from build123d import *

# Parameters (mm, degrees)
F0_R     = 2
F1_DEPTH = 0.5


with BuildPart() as f1:
    # F0 (on Front) → F1 (new body, symmetric)
    with BuildSketch(Plane.XZ):
        with BuildLine():
            Line((-25.05, -3.9878), (0, -3.9878))
            ThreePointArc((0, -3.9878), (3.9878, 0), (0, 3.9878))
            Line((0, 3.9878), (-25.05, 3.9878))
            Line((-25.05, 3.9878), (-25.05, -3.9878))
        make_face()
        with Locations((-19.0556, 0)):
            Circle(F0_R, mode=Mode.SUBTRACT)
        with Locations((-11.9944, 0)):
            Circle(F0_R, mode=Mode.SUBTRACT)
        Circle(F0_R, mode=Mode.SUBTRACT)
    extrude(amount=F1_DEPTH, both=True)


solid = f1.part
Geometry: final body of the model. Coordinates: model frame, mm. Round coordinates to 2 decimals unless told otherwise and drop trailing zeros. Loops run counter-clockwise (first coordinate to the right, second up) from the corner with the lowest first, then second, coordinate; pieces in that order, holes last. Notation, with made-up numbers: M 5.5,-2 L 64.5,-2 A21 ccw 64.5,31 Z; hole C -37,81 d10. An arc over 180 degrees is marked long. One line per question, with ' | ' between items.
(1) Cut plane C-C on z = -1.25. Return the cut outline in (x, y).
Check result:
outline: M -25.05,-0.5 L -20.62,-0.5 L -20.62,0.5 L -25.05,0.5 Z; M -17.49,-0.5 L -13.56,-0.5 L -13.56,0.5 L -17.49,0.5 Z; M -10.43,-0.5 L -1.56,-0.5 L -1.56,0.5 L -10.43,0.5 Z; M 1.56,-0.5 L 3.79,-0.5 L 3.79,0.5 L 1.56,0.5 Z
(2) Pull-direction query (X, two-part tool) for faces 1 (the cylindrical face through (0, 0, -2)), 2 (the flat face through (-13, 0, -3.988)), 3 (the cylindrical face through (3.987, -0.007, -0.088)); classes: +X half, -X half, draft (parallel to the pull), parting line (faces both ways), or undercut.
Check result:
face 1: undercut | face 2: draft | face 3: +X half
(3) Material intervals for line 1 along X through (y, z) = (-0.15, -0.5); line 2 along Z through (x, y) = (-19, -0.2); line 3 along Z through (x, y) = (-1, -0.1), sorted ascending. Write a range as from..to.
Check result:
line 1: x = -25.05..-20.99, -17.12..-13.93, -10.06..-1.94, 1.94..3.96 | line 2: z = -3.99..-2, 2..3.99 | line 3: z = -3.99..-1.73, 1.73..3.99
(4) Cut plane A-A on y = 0.2. Return the cut outline in (x, z), plus the area to 3 significant figures.
Check result:
outline: M -25.05,-3.99 L 0,-3.99 A3.99 ccw 0,3.99 L -25.05,3.99 Z; hole C -19.06,0 d4; hole C -11.99,0 d4; hole C 0,0 d4 | area: 187 mm2
(5) Cut plane B-B on z = 0. Return the cut outline in (x, y).
Check result:
outline: M -25.05,-0.5 L -21.06,-0.5 L -21.06,0.5 L -25.05,0.5 Z; M -17.06,-0.5 L -13.99,-0.5 L -13.99,0.5 L -17.06,0.5 Z; M -9.99,-0.5 L -2,-0.5 L -2,0.5 L -9.99,0.5 Z; M 2,-0.5 L 3.99,-0.5 L 3.99,0.5 L 2,0.5 Z
(6) Cut plane D-D on z = -2.75. Return the cut outline in (x, y), plus the area to 3 significant figures.
Check result:
outline: M -25.05,-0.5 L 2.89,-0.5 L 2.89,0.5 L -25.05,0.5 Z | area: 27.9 mm2
